Design review of the part built by this model. Coordinates are the model's own, in mm. Face numbers are marked on the shaded views. A direction names the side the tool comes from. Coordinates: 2 decimals unless noted, no trailing zeros. Write each loop counter-clockwise with the first axis right and the second up, starting at its lowest first coordinate (ties: lowest second). Pieces come first, ordered by that corner, then holes. Notation, with made-up numbers: M -21.75,1.25 L 17.25,1.25 A33 cw 17.25,31.25 Z; hole C 30,24.25 d1. An arc over 180 degrees is marked long. One line per question, with ' | ' between items.
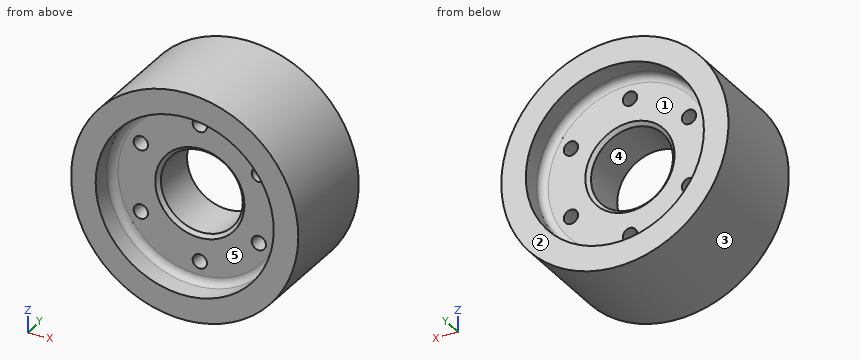
from build123d import *

# Parameters (mm, degrees)
SKETCH1_R              = 38.1
SKETCH1_R_2            = 14.3129
BOSS_EXTRUDE1_DEPTH    = 9.525
SKETCH2_R              = 39.6875
SKETCH2_R_2            = 31.115
BOSS_EXTRUDE2_DEPTH    = 19.05
F_10_CLEARANCE_HOLE1_D = 4.9784
CIRPATTERN1_COUNT      = 6
CHAMFER1_SIZE          = 1.27
FILLET2_R              = 2.54


with BuildPart() as part:
    # Sketch1 → Boss-Extrude1 (new body, symmetric)
    with BuildSketch(Plane(origin=(0, 0, 0), x_dir=(1, 0, 0), z_dir=(0, 1, 0))):
        Circle(SKETCH1_R)
        Circle(SKETCH1_R_2, mode=Mode.SUBTRACT)
    extrude(amount=BOSS_EXTRUDE1_DEPTH, both=True)

    # Sketch2 → Boss-Extrude2 (add, symmetric)
    with BuildSketch(Plane(origin=(0, 0, 0), x_dir=(1, 0, 0), z_dir=(0, 1, 0))):
        Circle(SKETCH2_R)
        Circle(SKETCH2_R_2, mode=Mode.SUBTRACT)
    extrude(amount=BOSS_EXTRUDE2_DEPTH, both=True)

    # #10 Clearance Hole1 (through all)
    with Locations(Plane(origin=(0, 9.525, 0), x_dir=(1, 0, 0), z_dir=(0, 1, 0))):
        with Locations((0, 23.8125)):
            f_10_clearance_hole1 = Hole(F_10_CLEARANCE_HOLE1_D / 2)

    # CirPattern1: #10 Clearance Hole1 ×6 about axis
    cirpattern1_axis = Axis((0, 0, 0), (0, 1, 0))
    for i in range(1, CIRPATTERN1_COUNT):
        add(f_10_clearance_hole1.rotate(cirpattern1_axis, i * 360 / CIRPATTERN1_COUNT), mode=Mode.SUBTRACT)

    # Chamfer1
    chamfer1_edges = [part.edges().sort_by_distance(p)[0] for p in [
        (-14.3129, -9.525, 0),
        (-14.3129, 9.525, 0),
    ]]
    chamfer(chamfer1_edges, length=CHAMFER1_SIZE)

    # Fillet2
    fillet2_edges = [part.edges().sort_by_distance(p)[0] for p in [
        (-31.115, 9.525, 0),
        (-31.115, -9.525, 0),
    ]]
    fillet(fillet2_edges, radius=FILLET2_R)


solid = part.part
1. Take a section at C-C (y = -16.5). Write out the cut boundary in (x, z) (1 decimal).
Answer sheet:
outline: C 0,0 d79.4; hole C 0,0 d62.2
2. Take a section at D-D (y = 2). Write out the cut boundary in (x, z) (1 decimal).
Answer sheet:
outline: C 0,0 d79.4; hole C -20.6,-11.9 d5; hole C -20.6,11.9 d5; hole C 0,0 d28.6; hole C 0,-23.8 d5; hole C 0,23.8 d5; hole C 20.6,-11.9 d5; hole C 20.6,11.9 d5
3. Tool access review of the marked faces 4 and 5: name each direction out of +Z, -Z, +X, -X, +Y, -Y from which nothing blocks a thin tool from reaching the whole face with its end or side.
Answer sheet:
face 4: +Y, -Y | face 5: -Y
4. Take a section at A-A (x = 0). Count the separate pieces of the cut face and the enclosed holes in it, then the cut area to 3 significant figures.
Answer sheet:
separate pieces: 4 | enclosed holes: 0 | area: 1,110 mm^2
5. Insertion check: pin 1 Ø10 at (y, z) = (5, 6.5) entering from +X; pin 2 Ø4 at (x, z) = (0, 23.81) entering from +Y; pin 3 Ø4 at (y, z) = (15, -19) entering from -X; pin 4 Ø1 at (x, y) = (8.5, 12) entering from -Z. Each pin has a flat end and moves straight along its axis. Give the tip position at first contact, or say it passes through.
Answer sheet:
pin 1: x = 39.66 | pin 2: through | pin 3: x = -35.86 | pin 4: z = -38.87
6. Draft analysis for pull direction Z (two halves, no side actions). For the marked faces 1, 2 and 3, state which applies: pulls with the +Z half, pulls with the -Z half, needs draft (parallel to the pull), parting line crosses it, or undercut.
Answer sheet:
face 1: undercut | face 2: needs draft | face 3: parting line crosses it
7. To check wall thickness, follow line 1 along Z through (x, y) = (0, 0); line 2 along X through (y, z) = (8.5, -10.5); line 3 along X through (y, z) = (5, -11). State the ranges of each line that lie inside material, in increasing order. Write a range as [from, to].
Answer sheet:
line 1: [-39.69, -26.3], [-21.32, -14.31], [14.31, 21.32], [26.3, 39.69] | line 2: [-38.27, -22.68], [-18.57, -10.08], [10.08, 18.57], [22.68, 38.27] | line 3: [-38.13, -22.94], [-18.3, -9.16], [9.16, 18.3], [22.94, 38.13]
